```python
from build123d import *

# Parameters (mm, degrees)
SKETCH1_W           = 406.4
SKETCH1_H           = 406.4
BOSS_EXTRUDE1_DEPTH = 6.35
SKETCH2_W           = 12.7
SKETCH2_H           = 12.7
BOSS_EXTRUDE2_DEPTH = 381
SKETCH3_W           = 406.4
SKETCH3_H           = 406.4
SKETCH3_W_2         = 381
SKETCH3_H_2         = 381
BOSS_EXTRUDE3_DEPTH = 6.35
SKETCH4_W           = 381
SKETCH4_H           = 228.6
BOSS_EXTRUDE4_DEPTH = 6.35
SKETCH6_W           = 381
SKETCH6_H           = 387.35
BOSS_EXTRUDE6_DEPTH = 3.175


with BuildPart() as part:
    # Sketch1 → Boss-Extrude1 (new body)
    with BuildSketch(Plane(origin=(0, 0, 0), x_dir=(1, 0, 0), z_dir=(0, 1, 0))):
        Rectangle(SKETCH1_W, SKETCH1_H)
    extrude(amount=BOSS_EXTRUDE1_DEPTH)

    # Sketch2 → Boss-Extrude2 (add)
    with BuildSketch(Plane(origin=(0, 6.35, 0), x_dir=(1, 0, 0), z_dir=(0, 1, 0))):
        with Locations((-196.85, 196.85)):
            Rectangle(SKETCH2_W, SKETCH2_H)
        with Locations((196.85, 196.85)):
            Rectangle(SKETCH2_W, SKETCH2_H)
        with Locations((196.85, -196.85)):
            Rectangle(SKETCH2_W, SKETCH2_H)
        with Locations((-196.85, -196.85)):
            Rectangle(SKETCH2_W, SKETCH2_H)
    extrude(amount=BOSS_EXTRUDE2_DEPTH)

    # Sketch3 → Boss-Extrude3 (add)
    with BuildSketch(Plane(origin=(0, 387.35, 0), x_dir=(1, 0, 0), z_dir=(0, 1, 0))):
        Rectangle(SKETCH3_W, SKETCH3_H)
        Rectangle(SKETCH3_W_2, SKETCH3_H_2, mode=Mode.SUBTRACT)
    extrude(amount=BOSS_EXTRUDE3_DEPTH)

    # Sketch4 → Boss-Extrude4 (add)
    with BuildSketch(Plane(origin=(0, 6.35, 0), x_dir=(1, 0, 0), z_dir=(0, 1, 0))):
        with Locations((0, -304.8)):
            Rectangle(SKETCH4_W, SKETCH4_H)
    extrude(amount=-BOSS_EXTRUDE4_DEPTH)

    # Sketch6 → Boss-Extrude6 (add)
    with BuildSketch(Plane.XY.offset(419.1)):
        with Locations((0, 193.675)):
            Rectangle(SKETCH6_W, SKETCH6_H)
    extrude(amount=BOSS_EXTRUDE6_DEPTH)


solid = part.part
```
For this review, take the finished solid that the model builds, in its own axes (mm). A direction names the side the tool comes from. Round coordinates to 2 decimals unless told otherwise and drop trailing zeros. Write each loop counter-clockwise with the first axis right and the second up, starting at its lowest first coordinate (ties: lowest second). Pieces come first, ordered by that corner, then holes. Notation, with made-up numbers: (4.5, 53.25) - (30.5, 53.25) arc R9 cw to (30.5, 70.25) - close; hole circle Ø10 at (2, 86). An arc over 180 degrees is marked (long way). Write each question's results on one line, items separated by ' | '.
Item 1: Take a section at C-C on x = 91.5. State the section outline as (y, z) points (3 decimals), then the cut area to 3 significant figures.
Calculated:
outline: (0, -203.2) - (6.35, -203.2) - (6.35, 419.1) - (387.35, 419.1) - (387.35, 422.275) - (0, 422.275) - close; (387.35, -203.2) - (393.7, -203.2) - (393.7, -190.5) - (387.35, -190.5) - close; (387.35, 190.5) - (393.7, 190.5) - (393.7, 203.2) - (387.35, 203.2) - close | area: 5,340 mm^2
Item 2: Take a section at A-A on y = 108.5. State the section outline as (x, z) points (3 decimals), then the cut area to 3 significant figures.
Calculated:
outline: (-203.2, -203.2) - (-190.5, -203.2) - (-190.5, -190.5) - (-203.2, -190.5) - close; (-203.2, 190.5) - (-190.5, 190.5) - (-190.5, 203.2) - (-203.2, 203.2) - close; (-190.5, 419.1) - (190.5, 419.1) - (190.5, 422.275) - (-190.5, 422.275) - close; (190.5, -203.2) - (203.2, -203.2) - (203.2, -190.5) - (190.5, -190.5) - close; (190.5, 190.5) - (203.2, 190.5) - (203.2, 203.2) - (190.5, 203.2) - close | area: 1,850 mm^2
Item 3: Draft analysis for pull direction Y (two halves, no side actions). For faces 1 (the face through (-16, 393.7, 195)), 2 (the face through (-197, 194, 190.5)), 3 (the face through (-3, 200, 419.1)), state which applies: pulls with the +Y half, pulls with the -Y half, needs draft (parallel to the pull), parting line crosses it, or undercut.
Calculated:
face 1: pulls with the +Y half | face 2: undercut | face 3: needs draft
Item 4: Take a section at B-B on z = 30. State the section outline as (x, y) points, then the cut area to 3 significant figures.
Calculated:
outline: (-203.2, 0) - (203.2, 0) - (203.2, 6.35) - (-203.2, 6.35) - close; (-203.2, 387.35) - (-190.5, 387.35) - (-190.5, 393.7) - (-203.2, 393.7) - close; (190.5, 387.35) - (203.2, 387.35) - (203.2, 393.7) - (190.5, 393.7) - close | area: 2,740 mm^2
Item 5: Take a section at D-D on z = 232.5. State the section outline as (x, y) points, then the cut area to 3 significant figures.
Calculated:
outline: (-190.5, 0) - (190.5, 0) - (190.5, 6.35) - (-190.5, 6.35) - close | area: 2,420 mm^2
Item 6: For pin 1 (4 mm diameter, centred on x = -11, z = -117, fed in from +Y); pin 2 (6.5 mm diameter, centred on x = 197, y = 218.5, fed in from +Z); pin 3 (2.5 mm diameter, centred on x = 56.5, z = 421.5, fed in from +Y), all flat-tipped, find the tip position at first contact; note any pin that passes through.
Calculated:
pin 1: stops at y = 6.35 | pin 2: stops at z = 203.2 | pin 3: stops at y = 387.35
Item 7: To check wall thickness, follow line 1 along X through (y, z) = (58.5, 201.5); line 2 along Y through (x, z) = (-133.5, 331.5); line 3 along Z through (x, y) = (109.5, 345) (3 decimals). State the ranges of each line that lie inside material, in increasing order. Write a range as from..to.
Calculated:
line 1: x = -203.2..-190.5, 190.5..203.2 | line 2: y = 0..6.35 | line 3: z = 419.1..422.275
Item 8: For faces 4 (the face through (-197, 194, -190.5)), 5 (the face through (190.5, 6, 312)), 6 (the face through (203.2, 196, -195)), 7 (the face through (190.5, 194, 197)), list the 3-axis set-ups (+Z, -Z, +X, -X, +Y, -Y) from which the entire face can be reached by the end or side of a thin tool; tool diameter is ignored.
Calculated:
face 4: +X, -X | face 5: +Z, +X, +Y, -Y | face 6: +Z, -Z, +X, +Y, -Y | face 7: -Z
